Drawing for the job (mm, zero at the part's lowest x, y, z). Give positions to 0.01 mm unless a question says otherwise; leave off trailing zeros. Order: outer loops, then holes, each group sorted by start corner. A loop starts at its lowest first (then second) coordinate and runs counter-clockwise, first axis right, second up. Notation, with made-up numbers: (-29.5, -6) -> (-4.5, -6) arc R23 cw to (-4.5, 14) -> close; hole circle Ø4 at (-35, 41). An arc over 180 degrees is marked (long way). Use one line per item in the form item = value. Start each with the question number.
1) Cut at D-D, the plane z = 8. Give the cut face in (x, y).
2) Cut at A-A, the plane x = 12.5. Give the cut face in (y, z).
3) Cut at B-B, the plane z = 12.5. Give the cut face in (x, y), and give its area (3 significant figures).
4) Cut at C-C, the plane y = 0.5. State how many separate pieces and enclosed holes the cut face has, and give its area (3 significant figures).
5) Probe line 1 (Z direction, x = 12.5, y = 0.75); line 2 (Z direction, x = 21.5, y = 0.95) (1 decimal); line 3 (Z direction, x = 20.25, y = 0.35) (1 decimal). List the from-to ranges inside material, lowest first.
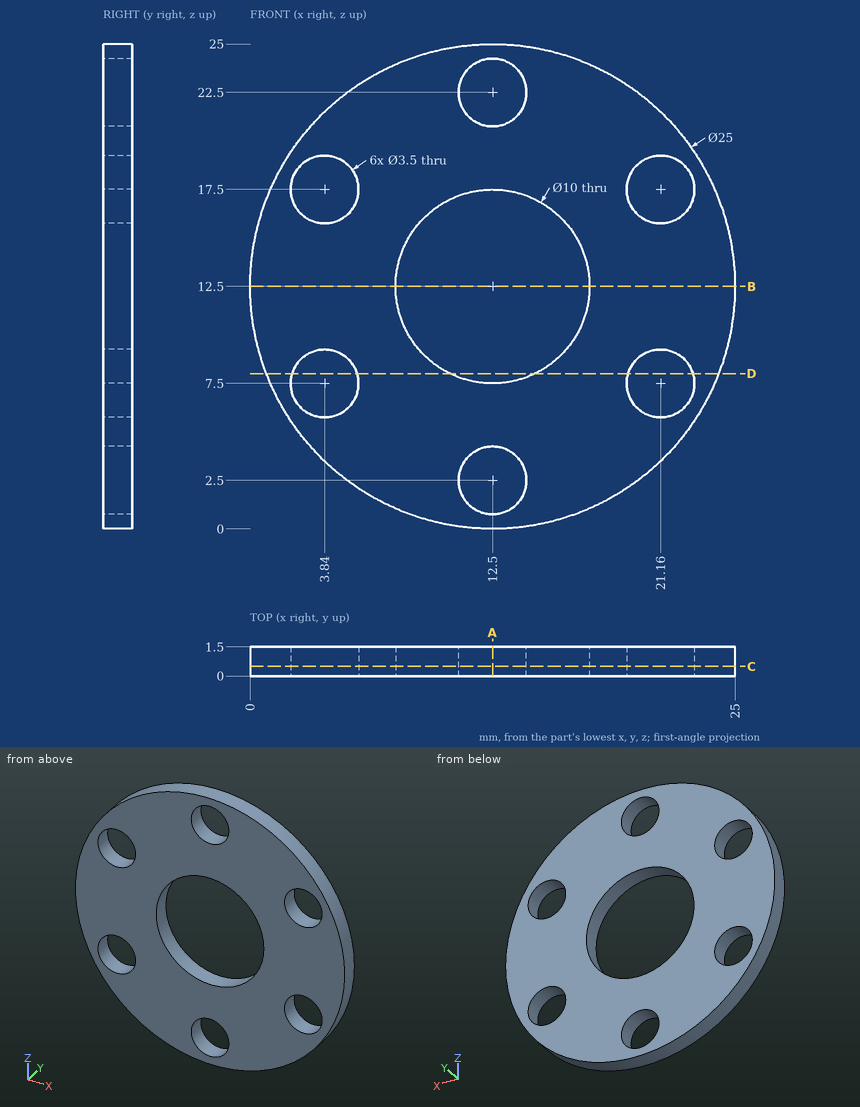
Result:
q1.outline = (0.84, 0) -> (2.16, 0) -> (2.16, 1.5) -> (0.84, 1.5) -> close; (5.52, 0) -> (10.32, 0) -> (10.32, 1.5) -> (5.52, 1.5) -> close; (14.68, 0) -> (19.48, 0) -> (19.48, 1.5) -> (14.68, 1.5) -> close; (22.84, 0) -> (24.16, 0) -> (24.16, 1.5) -> (22.84, 1.5) -> close
q2.outline = (0, 0) -> (1.5, 0) -> (1.5, 0.75) -> (0, 0.75) -> close; (0, 4.25) -> (1.5, 4.25) -> (1.5, 7.5) -> (0, 7.5) -> close; (0, 17.5) -> (1.5, 17.5) -> (1.5, 20.75) -> (0, 20.75) -> close; (0, 24.25) -> (1.5, 24.25) -> (1.5, 25) -> (0, 25) -> close
q3.outline = (0, 0) -> (7.5, 0) -> (7.5, 1.5) -> (0, 1.5) -> close; (17.5, 0) -> (25, 0) -> (25, 1.5) -> (17.5, 1.5) -> close
q3.area = 22.5 mm²
q4.separate_pieces = 1
q4.enclosed_holes = 7
q4.area = 355 mm²
q5.line_1 = 0 to 0.75, 4.25 to 7.5, 17.5 to 20.75, 24.25 to 25
q5.line_2 = 3.8 to 5.8, 9.2 to 15.8, 19.2 to 21.2
q5.line_3 = 2.7 to 6, 9 to 16, 19 to 22.3
